Part print with two shaded views. Sizes in mm from the minimum x, y, z corner. A direction names the side the tool comes from. Give positions to 0.01 mm unless a question says otherwise; leave off trailing zeros. Loops run counter-clockwise (first coordinate to the right, second up) from the corner with the lowest first, then second, coordinate; pieces in that order, holes last. Notation, with made-up numbers: M 74,88 L 131,88 A19 cw 131,123 Z; hole C 56.25,74 d1. An arc over 180 degrees is marked long. Answer in a Markdown table with one row per item.
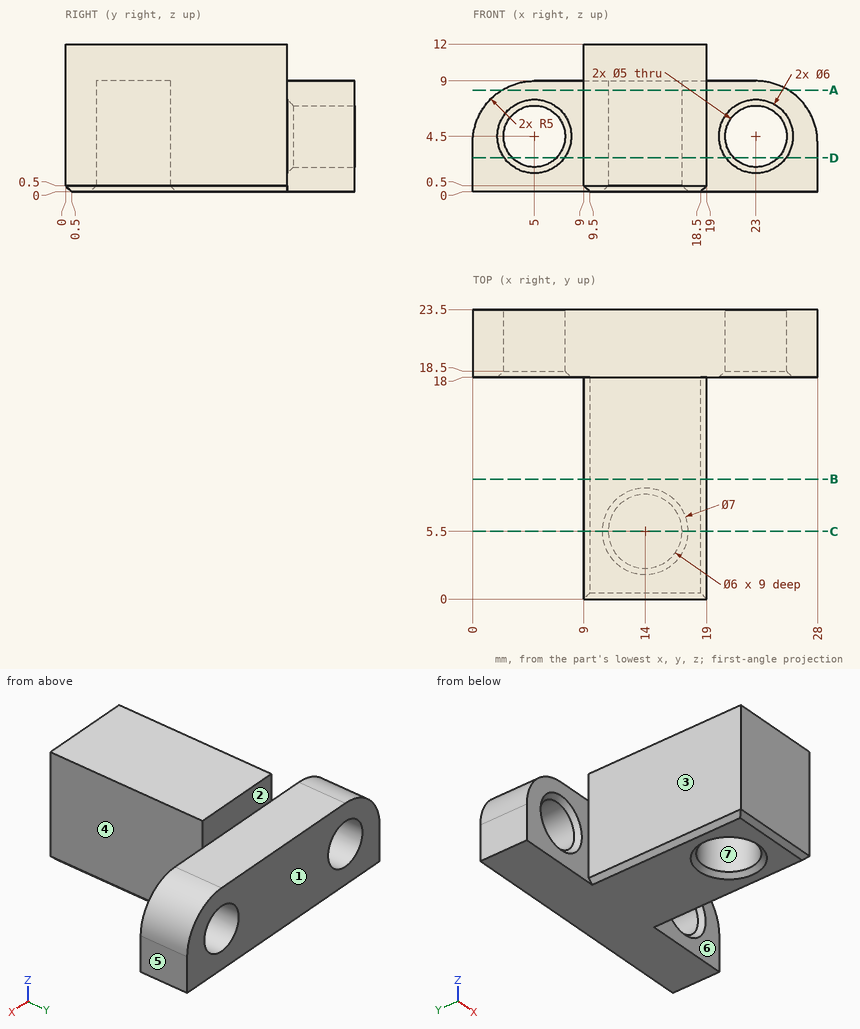
Q1. Drop flat-ended pins along their axis: pin 1 (3 mm diameter, centred on x = 5, z = 4.5, fed in from +Y); pin 2 (4 mm diameter, centred on y = 12.5, z = 3.5, fed in from -X); pin 3 (4.5 mm diameter, centred on x = 12, y = 21, fed in from +Z); pin 4 (4.5 mm diameter, centred on x = 4.5, z = 6, fed in from -Y). Give the stop position or say it passes through.
Reported:
| item | result |
|---|---|
| pin 1 | through |
| pin 2 | x = 9 |
| pin 3 | z = 9 |
| pin 4 | y = 18 |
Q2. Saw through at D-D (z = 2.75). Give the number of separate pieces and of enclosed holes in the cut face, and give its area (3 significant figures).
Reported:
| item | result |
|---|---|
| separate pieces | 3 |
| enclosed holes | 1 |
| area | 266 mm² |
Q3. Saw through at C-C (y = 5.5). Give the cut face in (x, z).
Reported:
| item | result |
|---|---|
| outline | M 9,0.5 L 9.5,0 L 10.5,0 L 11,0.5 L 11,9 L 17,9 L 17,0.5 L 17.5,0 L 18.5,0 L 19,0.5 L 19,12 L 9,12 Z |
Q4. Mould opens along X. For the marked faces 5, 6 and 7 say: released by +X, released by -X, zero draft, split by the parting line, or undercut.
Reported:
| item | result |
|---|---|
| face 5 | released by +X |
| face 6 | zero draft |
| face 7 | undercut |
Q5. 3-axis set-ups, long thin cutter, end or side, ignore diameter. For the marked faces 1, 2, 3 and 4: which of +Z, -Z, +X, -X, +Y, -Y reach the whole face in a straight line?
Reported:
| item | result |
|---|---|
| face 1 | +Z, -Z, +X, -X, +Y |
| face 2 | +Z, +X, -X, +Y |
| face 3 | +Z, -Z, -X, -Y |
| face 4 | +Z, -Z, +X, -Y |
Q6. Saw through at A-A (z = 8.25). Give the cut face in (x, y).
Reported:
| item | result |
|---|---|
| outline | M 2.37,18 L 9,18 L 9,0 L 19,0 L 19,18 L 25.63,18 L 25.63,23.5 L 2.37,23.5 Z; hole C 14,5.5 d6 |
Q7. Probe probe 1 along Z at (x, y) = (5, 21.2); probe 2 along Y at (x, z) = (14, 4.75); probe 3 along X at (y, z) = (13.25, 5.75). List the from-to ranges inside material, lowest first.
Reported:
| item | result |
|---|---|
| probe 1 | 0 to 2, 7 to 9 |
| probe 2 | 0 to 2.5, 8.5 to 23.5 |
| probe 3 | 9 to 19 |
Q8. Saw through at B-B (y = 9.75). Give the cut face in (x, z), and give its area (3 significant figures).
Reported:
| item | result |
|---|---|
| outline | M 9,0.5 L 9.5,0 L 18.5,0 L 19,0.5 L 19,12 L 9,12 Z |
| area | 120 mm² |
